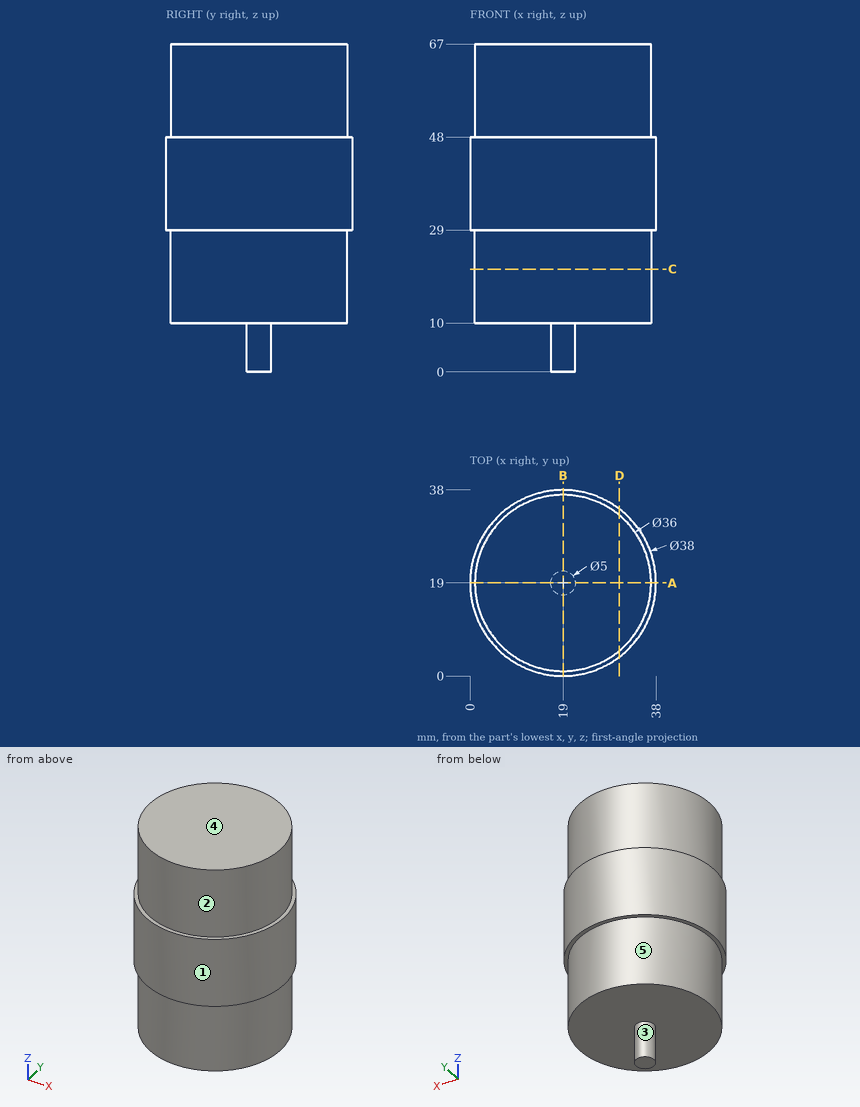
Can you work these out from the drawing? Everything is in mm from the part's minimum corner. A direction names the side the tool comes from. Give positions to 0.01 mm unless a question says otherwise; leave off trailing zeros. Order: outer loops, then holes, each group sorted by start corner. A loop starts at its lowest first (then second) coordinate and runs counter-clockwise, first axis right, second up.
1. Suppose I cut it at C-C (z = 21). List the corners of the cut face in (x, y) for me, plus the area to 3 significant figures.
2. I need wall thicknesses on L1, parallel to Z at x = 33, y = 7.5; L2, parallel to Z at x = 21, y = 32; L3, parallel to Y at x = 19, z = 58. Which ranges of each line are inside material? Lowest first, please.
3. Suppose I cut it at A-A (y = 19). List the corners of the cut face in (x, z) for me.
4. We'd pull the mould along X, two halves only. Please class the marked faces 4 and 5: pulls with the +X half, pulls with the -X half, needs draft (parallel to the pull), parting line crosses it, or undercut.
5. For the marked faces 1, 2 and 3, which set-ups out of +Z, -Z, +X, -X, +Y, -Y let a thin tool reach every point of the face, with its end or its side?
6. Will these pins go through, and if not, where does the flat tip stop? P1, Ø4, axis at y = 33.5, z = 48, coming from the -X side; P2, Ø10, axis at y = 31.5, z = 30, coming from the +X side; P3, Ø1.5, axis at x = 10.5, y = 12, coming from the -Z side.
7. Suppose I cut it at D-D (x = 30.5). List the corners of the cut face in (y, z) for me.
Solved:
1. outline: circle Ø36 at (19, 19)
1. area: 1,020 mm2
2. L1: z = 29 to 48
2. L2: z = 10 to 67
2. L3: y = 1 to 37
3. outline: (0, 29) - (1, 29) - (1, 10) - (16.5, 10) - (16.5, 0) - (21.5, 0) - (21.5, 10) - (37, 10) - (37, 29) - (38, 29) - (38, 48) - (37, 48) - (37, 67) - (1, 67) - (1, 48) - (0, 48) - close
4. face 4: needs draft
4. face 5: parting line crosses it
5. face 1: +Z, -Z
5. face 2: +Z
5. face 3: -Z
6. P1: stops at x = 4.69
6. P2: stops at x = 36.46
6. P3: stops at z = 10
7. outline: (3.88, 29) - (5.15, 29) - (5.15, 10) - (32.85, 10) - (32.85, 29) - (34.12, 29) - (34.12, 48) - (32.85, 48) - (32.85, 67) - (5.15, 67) - (5.15, 48) - (3.88, 48) - close
